Read the model definition and answer for the solid it produces. Units are mm, in the model's axes. Give positions to 0.01 mm unless a question says otherwise; leave off trailing zeros. Write each loop counter-clockwise with the first axis right and the second up, starting at its lowest first coordinate (ties: lowest second). Pieces come first, ordered by that corner, then holes. Notation, with made-up numbers: (7.25, 87) - (44.25, 87) arc R28 cw to (44.25, 118) - close; hole circle Ø2 at (-33, -17). An arc over 180 degrees is marked (long way). Use CSV: the item, a comma, the result in double quotes. Start each with the question number.
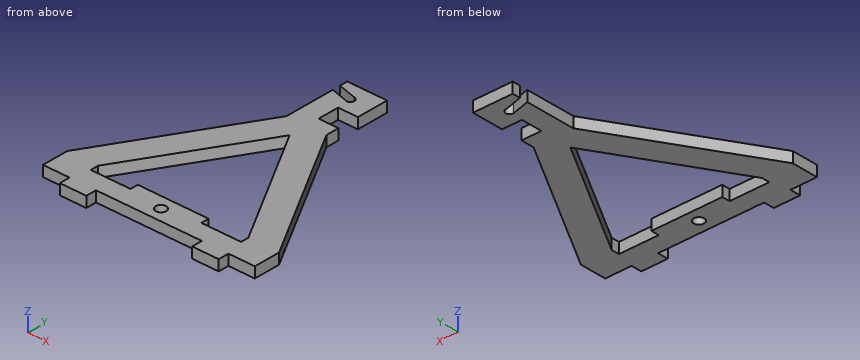
from build123d import *

# Parameters (mm, degrees)
SKETCH1_R           = 4
BOSS_EXTRUDE1_DEPTH = 8
SKETCH2_W           = 20
SKETCH2_H           = 8
BOSS_EXTRUDE2_DEPTH = 8
SKETCH4_W           = 15
SKETCH4_H           = 16
CUT_EXTRUDE1_DEPTH  = 10
SKETCH5_W           = 30
SKETCH5_H           = 6
CUT_EXTRUDE2_DEPTH  = 8
CUT_EXTRUDE4_DEPTH  = 198.139544486


with BuildPart() as part:
    # Sketch1 → Boss-Extrude1 (new body)
    with BuildSketch(Plane.XY):
        Polygon((-80, 0), (80, 0), (80, 20), (15, 130), (15, 180), (-15, 180), (-15, 130), (-80, 20), align=None)
        with Locations((0, 10)):
            Circle(SKETCH1_R, mode=Mode.SUBTRACT)
        Polygon((-56.769213929, 20), (0, 116.070977418), (56.769213929, 20), align=None, mode=Mode.SUBTRACT)
    extrude(amount=BOSS_EXTRUDE1_DEPTH)

    # Sketch2 → Boss-Extrude2 (add)
    with BuildSketch(Plane.XZ):
        with Locations((-50, 4)):
            Rectangle(SKETCH2_W, SKETCH2_H)
    boss_extrude2 = extrude(amount=BOSS_EXTRUDE2_DEPTH)

    # Mirror1: Boss-Extrude2 across plane
    add(boss_extrude2.mirror(Plane(origin=(0, 0, 0), x_dir=(0, 0, 1), z_dir=(1, 0, 0))))

    # Sketch4 → Cut-Extrude1 (cut)
    with BuildSketch(Plane.XY.offset(8)):
        with Locations((7.5, 148)):
            Rectangle(SKETCH4_W, SKETCH4_H)
    extrude(amount=-CUT_EXTRUDE1_DEPTH, mode=Mode.SUBTRACT)

    # Sketch5 → Cut-Extrude2 (cut)
    with BuildSketch(Plane.XY.offset(8)):
        with Locations((-41.769213929, 17)):
            Rectangle(SKETCH5_W, SKETCH5_H)
    cut_extrude2 = extrude(amount=-CUT_EXTRUDE2_DEPTH, mode=Mode.SUBTRACT)

    # Mirror2: Cut-Extrude2 across plane
    add(cut_extrude2.mirror(Plane(origin=(0, 0, 0), x_dir=(0, 0, 1), z_dir=(1, 0, 0))), mode=Mode.SUBTRACT)

    # Sketch7 → Cut-Extrude4 (cut, through all)
    with BuildSketch(Plane.XY.offset(8)):
        with BuildLine():
            Line((-15, 174), (-1, 170.248711306))
            ThreePointArc((-1, 170.248711306), (2, 167.248711306), (-1, 164.248711306))
            Line((-1, 164.248711306), (-15, 168))
            Line((-15, 168), (-15, 174))
        make_face()
    extrude(amount=-CUT_EXTRUDE4_DEPTH, mode=Mode.SUBTRACT)


solid = part.part
(1) Consider probe 1 along X at (y, z) = (19, 5.5); probe 2 along Y at (x, z) = (7.5, 4); probe 3 along X at (y, z) = (75.5, 1.5). Determine where each line is inside the solid, lowest interval first.
(2) Given P1, Ø4, axis at y = -4, z = 5.5, coming from the +X side; P2, Ø3, axis at y = 178.5, z = 3.5, coming from the -X side; P3, Ø4, axis at x = -27, z = 2, coming from the -Y side, each flat-ended and moving along its own axis, determine where each tip first touches the part or whether it passes through.
(3) The part is cut by section B-B on y = 10. Write down the section's boundary in (x, z).
(4) The part is cut by section C-C on x = -17. Write down the section's boundary in (y, z), plus the area to 3 significant figures.
(5) The part is cut by section A-A on z = 4. Give the number of separate pieces and of enclosed holes in the cut face, plus the area to 3 significant figures.
Reported:
1,probe 1,"-80 to -56.77, -26.77 to 26.77, 56.77 to 80"
1,probe 2,"0 to 20, 103.38 to 140, 156 to 180"
1,probe 3,"-47.2 to -23.97, 23.97 to 47.2"
2,P1,"x = 60"
2,P2,"x = -15"
2,P3,"y = 0"
3,outline,"(-80, 0) - (-4, 0) - (-4, 8) - (-80, 8) - close; (4, 0) - (80, 0) - (80, 8) - (4, 8) - close"
4,outline,"(0, 0) - (20, 0) - (20, 8) - (0, 8) - close; (87.3, 0) - (126.62, 0) - (126.62, 8) - (87.3, 8) - close"
4,area,"475 mm²"
5,separate pieces,"1"
5,enclosed holes,"2"
5,area,"9,270 mm²"
